from build123d import *

# Parameters (mm, degrees)
EXTRUDE_1_DEPTH     = 50
SKETCH_2_R          = 1.75
CUT_EXTRUDE_1_DEPTH = 85.787970845
CUT_EXTRUDE_2_REACH = 86.788
SKETCH_3_R          = 1.75


with BuildPart() as part:
    # 草图1 → 凸台-拉伸1 (new body)
    with BuildSketch(Plane(origin=(0, 0, 0), x_dir=(1, 0, 0), z_dir=(0, 1, 0))):
        Polygon((0, 0), (30, 0), (30, 60), (33, 60), (33, -3), (0, -3), align=None)
    extrude(amount=EXTRUDE_1_DEPTH)

    # 草图2 → 切除-拉伸1 (cut, through all)
    with BuildSketch(Plane(origin=(0, 0, 0), x_dir=(-1, 0, 0), z_dir=(0, 0, -1))):
        with Locations((-22, 6)):
            Circle(SKETCH_2_R)
        with Locations((-22, 44)):
            Circle(SKETCH_2_R)
        with Locations((-5, 44)):
            Circle(SKETCH_2_R)
        with Locations((-5, 6)):
            Circle(SKETCH_2_R)
    extrude(amount=-CUT_EXTRUDE_1_DEPTH, mode=Mode.SUBTRACT)

    # 草图3 → 切除-拉伸2 (cut, up to next)
    with BuildSketch(Plane(origin=(33, 0, 0), x_dir=(0, 0, -1), z_dir=(1, 0, 0)), mode=Mode.PRIVATE) as cut_extrude_2_sk1:
        with Locations((55, 35)):
            Circle(SKETCH_3_R)
    cut_extrude_2_tool1 = extrude(cut_extrude_2_sk1.sketch, amount=-CUT_EXTRUDE_2_REACH, mode=Mode.PRIVATE) & part.part
    # 草图3 → 切除-拉伸2 (cut, up to next)
    with BuildSketch(Plane(origin=(33, 0, 0), x_dir=(0, 0, -1), z_dir=(1, 0, 0)), mode=Mode.PRIVATE) as cut_extrude_2_sk2:
        with Locations((55, 15)):
            Circle(SKETCH_3_R)
    cut_extrude_2_tool2 = extrude(cut_extrude_2_sk2.sketch, amount=-CUT_EXTRUDE_2_REACH, mode=Mode.PRIVATE) & part.part
    # 草图3 → 切除-拉伸2 (cut, up to next)
    with BuildSketch(Plane(origin=(33, 0, 0), x_dir=(0, 0, -1), z_dir=(1, 0, 0)), mode=Mode.PRIVATE) as cut_extrude_2_sk3:
        with Locations((35, 35)):
            Circle(SKETCH_3_R)
    cut_extrude_2_tool3 = extrude(cut_extrude_2_sk3.sketch, amount=-CUT_EXTRUDE_2_REACH, mode=Mode.PRIVATE) & part.part
    # 草图3 → 切除-拉伸2 (cut, up to next)
    with BuildSketch(Plane(origin=(33, 0, 0), x_dir=(0, 0, -1), z_dir=(1, 0, 0)), mode=Mode.PRIVATE) as cut_extrude_2_sk4:
        with Locations((35, 15)):
            Circle(SKETCH_3_R)
    cut_extrude_2_tool4 = extrude(cut_extrude_2_sk4.sketch, amount=-CUT_EXTRUDE_2_REACH, mode=Mode.PRIVATE) & part.part
    add(cut_extrude_2_tool1.solids().sort_by_distance((33, 35, -55))[0], mode=Mode.SUBTRACT)
    add(cut_extrude_2_tool2.solids().sort_by_distance((33, 15, -55))[0], mode=Mode.SUBTRACT)
    add(cut_extrude_2_tool3.solids().sort_by_distance((33, 35, -35))[0], mode=Mode.SUBTRACT)
    add(cut_extrude_2_tool4.solids().sort_by_distance((33, 15, -35))[0], mode=Mode.SUBTRACT)


solid = part.part
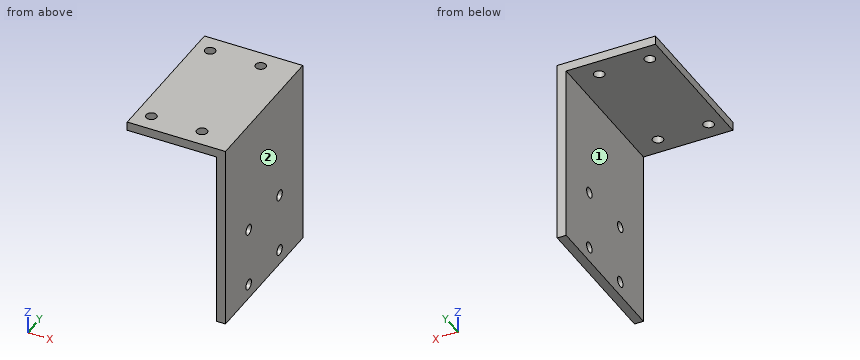
Build history of the part. All positions in model axes, mm. Face numbers are marked on the shaded views. A direction names the side the tool comes from. Round coordinates to 2 decimals unless told otherwise and drop trailing zeros. Write each loop counter-clockwise with the first axis right and the second up, starting at its lowest first coordinate (ties: lowest second). Pieces come first, ordered by that corner, then holes. Notation, with made-up numbers: (-27, 8.25) - (16, 8.25) arc R36 cw to (16, 44.25) - close; hole circle Ø11 at (40.5, -29.5). An arc over 180 degrees is marked (long way). One line per question, with ' | ' between items.
1. Drop flat-ended pins along their axis: pin 1 Ø5 at (y, z) = (12, -12.5) entering from -X; pin 2 Ø9 at (x, y) = (20.5, 25) entering from -Z. Give the stop position or say it passes through.
Results are:
pin 1: x = 30 | pin 2: z = 0
2. Band-saw the part on D-D, the plane y = 24.5. Write the cut outline in (x, z).
Results are:
outline: (0, 0) - (30, 0) - (30, -60) - (33, -60) - (33, 3) - (0, 3) - close
3. Drill centre lines: line 1 along Y through (x, z) = (32.3, -55); line 2 along Y through (x, z) = (5, 0.9); line 3 along X through (y, z) = (4, -30). Where is each one in solid material? Low to high. Write a range as from..to.
Results are:
line 1: 0..13.25, 16.75..33.25, 36.75..50 | line 2: 0..4.25, 7.75..42.25, 45.75..50 | line 3: 30..33
4. Tool access for the marked faces 1 and 2: list every direction of +Z, -Z, +X, -X, +Y, -Y with a clear straight run to the whole face (end or side of a thin tool).
Results are:
face 1: -Z, -X, +Y, -Y | face 2: +Z, -Z, +X, +Y, -Y
5. Band-saw the part on A-A, the plane z = -35. Write the cut outline in (x, y).
Results are:
outline: (30, 0) - (33, 0) - (33, 13.25) - (30, 13.25) - close; (30, 16.75) - (33, 16.75) - (33, 33.25) - (30, 33.25) - close; (30, 36.75) - (33, 36.75) - (33, 50) - (30, 50) - close
6. Band-saw the part on C-C, the plane x = 5. Write the cut outline in (y, z), and give its area (3 significant figures).
Results are:
outline: (0, 0) - (4.25, 0) - (4.25, 3) - (0, 3) - close; (7.75, 0) - (42.25, 0) - (42.25, 3) - (7.75, 3) - close; (45.75, 0) - (50, 0) - (50, 3) - (45.75, 3) - close | area: 129 mm^2
7. Band-saw the part on B-B, the plane y = 15. Write the cut outline in (x, z).
Results are:
outline: (0, 0) - (30, 0) - (30, -33.25) - (33, -33.25) - (33, 3) - (0, 3) - close; (30, -60) - (33, -60) - (33, -56.75) - (30, -56.75) - close; (30, -53.25) - (33, -53.25) - (33, -36.75) - (30, -36.75) - close
